from build123d import *

# Parameters (mm, degrees)
F0_W     = 38.1
F0_H     = 17.78
F1_DEPTH = 5.08
F2_T     = -5.08
F3_T     = -2.54


with BuildPart() as f1:
    # F0 (on Front) → F1 (new body)
    with BuildSketch(Plane.XZ):
        with Locations((0.816431, -2.540001)):
            Rectangle(F0_W, F0_H)
    extrude(amount=F1_DEPTH)

    # F2
    f2_openings = [f1.faces().sort_by_distance(p)[0] for p in [
        (0.816431, 0, -2.540001),
    ]]
    offset(amount=F2_T, openings=f2_openings)

    # F3
    f3_openings = [f1.faces().sort_by_distance(p)[0] for p in [
        (0.816431, 0, -2.540001),
    ]]
    offset(amount=F3_T, openings=f3_openings)


solid = f1.part
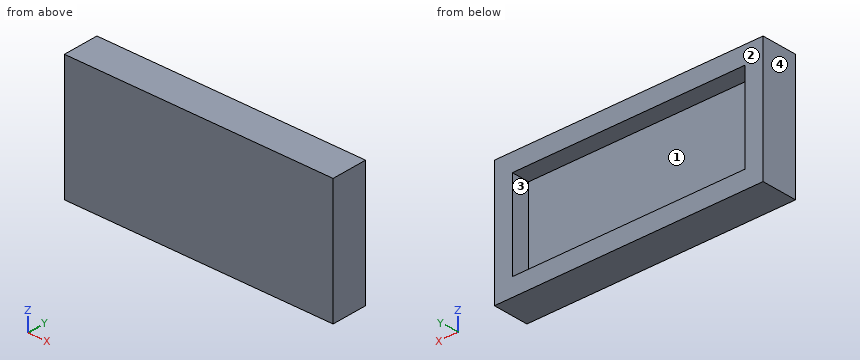
Geometry: final body of the model. Coordinates: model frame, mm. Face numbers are marked on the shaded views. Give positions to 0.01 mm unless a question says otherwise; leave off trailing zeros. Loops run counter-clockwise (first coordinate to the right, second up) from the corner with the lowest first, then second, coordinate; pieces in that order, holes last. Notation, with made-up numbers: M 51,-23.5 L 108,-23.5 A37 cw 108,14.5 Z; hole C -18,81 d10. An arc over 180 degrees is marked long. Put each result on its own line as item: value.
1) Cut plane C-C, the plane z = -8. Return the cut outline in (x, y).
Computed values:
outline: M -18.23,-5.08 L 19.87,-5.08 L 19.87,0 L 17.33,0 L 17.33,-2.54 L -15.69,-2.54 L -15.69,0 L -18.23,0 Z
2) Material intervals for L1, parallel to X at y = -1.75, z = -5.25; L2, parallel to Z at x = 8, y = -1.4; L3, parallel to Y at x = 3, z = 1.5, sorted ascending. Write a range as from..to.
Computed values:
L1: x = -18.23..-15.69, 17.33..19.87
L2: z = -11.43..-8.89, 3.81..6.35
L3: y = -5.08..-2.54
3) Cut plane A-A, the plane y = -1.3. Return the cut outline in (x, z).
Computed values:
outline: M -18.23,-11.43 L 19.87,-11.43 L 19.87,6.35 L -18.23,6.35 Z; hole M -15.69,-8.89 L 17.33,-8.89 L 17.33,3.81 L -15.69,3.81 Z
4) Cut plane B-B, the plane x = 5. Return the cut outline in (y, z).
Computed values:
outline: M -5.08,-11.43 L 0,-11.43 L 0,-8.89 L -2.54,-8.89 L -2.54,3.81 L 0,3.81 L 0,6.35 L -5.08,6.35 Z
5) First-contact query: P1, Ø4, axis at x = 0, z = -0.5, coming from the +Y side. Flat tip, straight axial feed; report the tip coordinate or a pass-through.
Computed values:
P1: stops at y = -2.54
6) Mould query, pull axis X, two halves, no side actions, for the marked faces 1, 2, 3 and 4. Classes: released by +X, released by -X, zero draft, split by the parting line, or undercut.
Computed values:
face 1: undercut
face 2: zero draft
face 3: undercut
face 4: released by -X
